```python
from build123d import *

# Parameters (mm, degrees)
SKETCH1_R           = 8.4
BOSS_EXTRUDE1_DEPTH = 34
SKETCH2_R           = 3.5
BOSS_EXTRUDE2_DEPTH = 1
FILLET1_R           = 1
FILLET2_R           = 0.4


with BuildPart() as part:
    # Sketch1 → Boss-Extrude1 (new body)
    with BuildSketch(Plane.XY):
        Circle(SKETCH1_R)
    extrude(amount=BOSS_EXTRUDE1_DEPTH)

    # Sketch2 → Boss-Extrude2 (add)
    with BuildSketch(Plane.XY.offset(34)):
        Circle(SKETCH2_R)
    extrude(amount=BOSS_EXTRUDE2_DEPTH)

    # Fillet1
    fillet1_edges = [part.edges().sort_by_distance(p)[0] for p in [
        (-8.4, 0, 0),
        (-8.4, 0, 34),
    ]]
    fillet(fillet1_edges, radius=FILLET1_R)

    # Fillet2
    fillet2_edges = [part.edges().sort_by_distance(p)[0] for p in [
        (-3.5, 0, 34),
        (-3.5, 0, 35),
    ]]
    fillet(fillet2_edges, radius=FILLET2_R)


solid = part.part
```
Part model, mm, in its own coordinate system. A direction names the side the tool comes from. Coordinates: 2 decimals unless noted, no trailing zeros. Order: outer loops, then holes, each group sorted by start corner. A loop starts at its lowest first (then second) coordinate and runs counter-clockwise, first axis right, second up. Notation, with made-up numbers: (-37, 47.5) -> (20, 47.5) arc R25 cw to (20, 78.5) -> close; hole circle Ø8 at (66, -30.5). An arc over 180 degrees is marked (long way). Put each result on its own line as item: value. Start each with the question number.
(1) Probe line 1 along Z through (x, y) = (-4.5, -1.75); line 2 along Y through (x, z) = (-5, 28.5); line 3 along Z through (x, y) = (-1, 3). List the from-to ranges inside material, lowest first. Write a range as [from, to].
(2) Which spindle directions (+Z, -Z, +X, -X, +Y, -Y) get a long thin tool onto all of the face, cutting with end or side? Do faces 1 (the face through (3, -3, 34)), 2 (the face through (0, 0, 35)). Say none if no direction does.
(3) Band-saw the part on C-C (z = 7). Give the cut face in (x, y).
(4) Band-saw the part on A-A (y = 0). Give the cut face in (x, z).
(5) Pin check, flat tips, straight feed: pin 1 Ø4 at (y, z) = (3.5, 30) entering from -X (3 decimals); pin 2 Ø3 at (x, z) = (3.5, 11.5) entering from -Y; pin 3 Ø4 at (x, z) = (-4.5, 4) entering from +Y. Stop position of each tip, or through.
Determined:
1. line 1: z = [0, 34]
1. line 2: y = [-6.75, 6.75]
1. line 3: z = [0, 35]
2. face 1: +Z
2. face 2: +Z, +X, -X, +Y, -Y
3. outline: circle Ø16.8 at (0, 0)
4. outline: (-8.4, 1) arc R1 ccw to (-7.4, 0) -> (7.4, 0) arc R1 ccw to (8.4, 1) -> (8.4, 33) arc R1 ccw to (7.4, 34) -> (3.9, 34) arc R0.4 cw to (3.5, 34.4) -> (3.5, 34.6) arc R0.4 ccw to (3.1, 35) -> (-3.1, 35) arc R0.4 ccw to (-3.5, 34.6) -> (-3.5, 34.4) arc R0.4 cw to (-3.9, 34) -> (-7.4, 34) arc R1 ccw to (-8.4, 33) -> close
5. pin 1: stops at x = -8.265
5. pin 2: stops at y = -8.16
5. pin 3: stops at y = 8.02
